Input: dimensioned drawing with shaded views. Units: mm. Origin: part minimum x, y, z. Give positions to 0.01 mm unless a question says otherwise; leave off trailing zeros. Write each loop counter-clockwise with the first axis right and the second up, starting at its lowest first coordinate (ties: lowest second). Pieces come first, ordered by that corner, then holes.
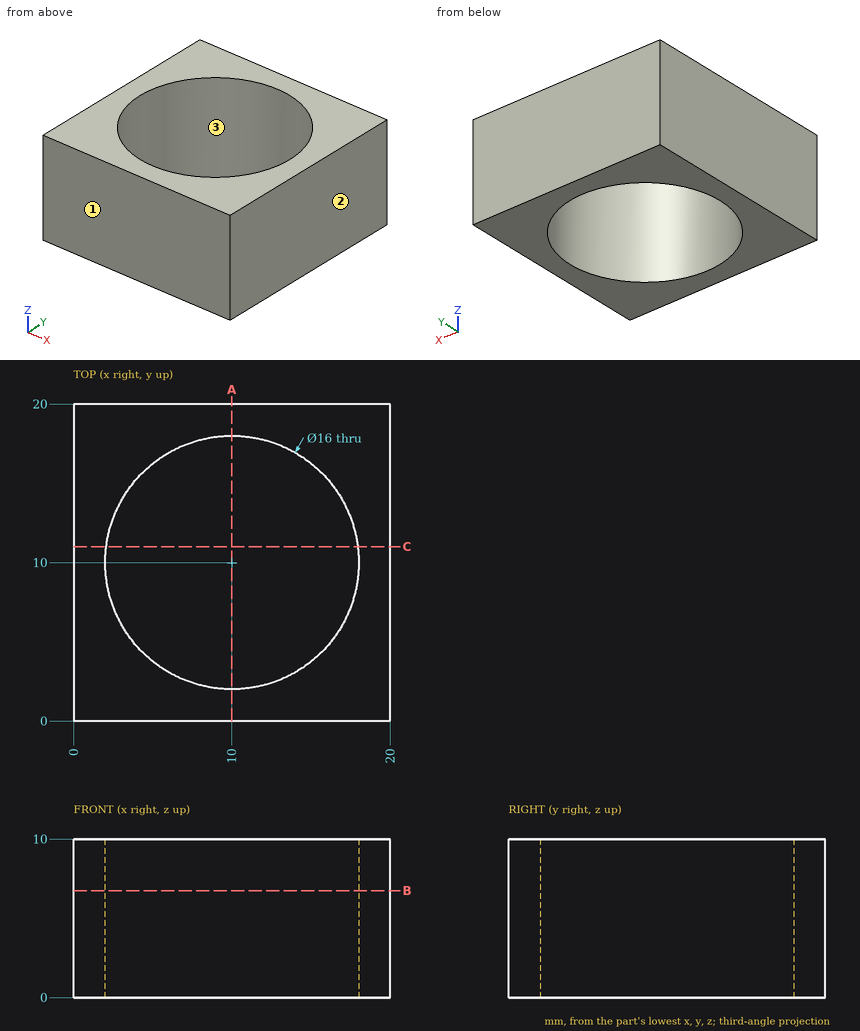
1. Cut plane C-C, the plane y = 11. Return the cut outline in (x, z).
2. Line query: L1, parallel to Y at x = 10, z = 7.5; L2, parallel to X at y = 4.5, z = 4.75; L3, parallel to X at y = 14.75, z = 7.5. Output: solid intervals per line, ascending.
3. Cut plane A-A, the plane x = 10. Return the cut outline in (y, z), then the cut area to 3 significant figures.
4. Mould query, pull axis Y, two halves, no side actions, for the marked faces 1, 2 and 3. Classes: +Y half, -Y half, draft (parallel to the pull), parting line (faces both ways), or undercut.
5. Cut plane B-B, the plane z = 6.75. Return the cut outline in (x, y), then the cut area to 3 significant figures.
6. Contact query for a flat-ended pin moving along its axis: P1, Ø5, axis at x = 7.5, y = 13.5, coming from the +Z side (3 decimals). Output: stop coordinate, or through.
Response values:
1. outline: (0, 0) - (2.06, 0) - (2.06, 10) - (0, 10) - close; (17.94, 0) - (20, 0) - (20, 10) - (17.94, 10) - close
2. L1: y = 0 to 2, 18 to 20
2. L2: x = 0 to 4.19, 15.81 to 20
2. L3: x = 0 to 3.56, 16.44 to 20
3. outline: (0, 0) - (2, 0) - (2, 10) - (0, 10) - close; (18, 0) - (20, 0) - (20, 10) - (18, 10) - close
3. area: 40.0 mm2
4. face 1: -Y half
4. face 2: draft
4. face 3: undercut
5. outline: (0, 0) - (20, 0) - (20, 20) - (0, 20) - close; hole circle Ø16 at (10, 10)
5. area: 199 mm2
6. P1: passes through
